Can you work these out from the model? Positions are in its coordinate system, mm. A direction names the side the tool comes from. Coordinates: 2 decimals unless noted, no trailing zeros. Order: outer loops, then holes, each group sorted by start corner. A loop starts at its lowest first (then second) coordinate and runs counter-clockwise, first axis right, second up. Notation, with made-up numbers: (13.5, 12) -> (24.5, 12) arc R14 cw to (24.5, 25) -> close; hole circle Ø10 at (38, 40). An arc over 180 degrees is marked (long way). Use a Markdown table: item, result. Add a question column.
1. For faces 1 (the flat face through (6.4, -3.64, 3.92)), 2 (the conical face through (0.02, 4.89, 4.49)), 3 (the conical face through (-0.02, 4.89, 1.49)), which set-ups out of +Z, -Z, +X, -X, +Y, -Y let a thin tool reach every point of the face, with its end or its side?
2. For pin 1 Ø5 at (y, z) = (-4, 16.5) entering from +X; pin 2 Ø1.5 at (y, z) = (5, 9.5) entering from -X; pin 3 Ø1 at (x, y) = (-1, 0.5) entering from -Z; pin 4 Ø5 at (x, y) = (2.5, -3.5) entering from -Z, each with a flat end and sliding along its axis, tell me the tip position at first contact or that it passes through.
3. We'd pull the mould along Y, two halves only. Please class faces 4 (the conical face through (0.02, 4.89, 2.99)), 5 (the cylindrical face through (-3.988, 6.935, 3.749)), 6 (the cylindrical face through (-8, 0, 4)), 7 (the conical face through (0.02, 4.91, 4.97)): pulls with the +Y half, pulls with the -Y half, needs draft (parallel to the pull), parting line crosses it, or undercut.
4. If I drill on line 1 along X through (y, z) = (0, 5.75); line 2 along Z through (x, y) = (-4.75, 0.5); line 3 along X through (y, z) = (0, 2.65), over which ranges is the centre line in solid material (lowest first)? Write a range as from..to.
5. Suppose I cut it at B-B, the plane z = 12.5. List the corners of the cut face in (x, y) for me, then the cut area to 3 significant figures.
6. Suppose I cut it at A-A, the plane z = 5.5. List the corners of the cut face in (x, y) for me.
```python
from build123d import *

# Parameters (mm, degrees)
SKETCH001_R         = 14.291544
POCKET_DEPTH        = 24.501
REVOLUTION001_ANGLE = 30
REVOLUTION002_ANGLE = 30
REVOLUTION003_ANGLE = 30
REVOLUTION004_ANGLE = 30


with BuildPart() as part:
    # Sketch → Revolution (revolve)
    with BuildSketch(Plane.XZ):
        with BuildLine():
            Line((-5.3, 0), (-5.3, 6))
            ThreePointArc((-5.3, 6), (-4.244457, 6.413224), (-3.75, 7.433241))
            Line((-3.75, 7.433241), (-3, 17))
            Line((-3, 17), (-1.75, 20.5))
            Line((-1.75, 20.5), (-1.25, 20.5))
            Line((-1.25, 20.5), (-0.4, 24.5))
            Line((-0.4, 24.5), (-0.6, 24.5))
            Line((-5.526565, 16.862743), (-0.6, 24.5))
            Line((-5.526565, 16.862743), (-6.174059, 8.578152))
            Line((-6.174059, 8.578152), (-8, 7.60349))
            Line((-8, 7.60349), (-8, 0))
            Line((-5.3, 0), (-8, 0))
        make_face()
    revolve(axis=Axis((0, 0, 0), (0, 0, 1)))

    # Sketch001 (on Face12 of Revolution) → Pocket (cut, through all)
    with BuildSketch(Plane(origin=(0, 0, 0), x_dir=(1, 0, 0), z_dir=(0, 0, -1))):
        Circle(SKETCH001_R)
        Polygon((8.5, 0), (4.25, 7.361216), (-4.25, 7.361216), (-8.5, 0), (-4.25, -7.361216), (4.25, -7.361216), align=None, mode=Mode.SUBTRACT)
    extrude(amount=-POCKET_DEPTH, mode=Mode.SUBTRACT)

    # Sketch002 → Revolution001 (revolve, symmetric)
    with BuildSketch(Plane.XZ) as revolution001_sk:
        Polygon((-5.5, 0), (-4.5, 0.6), (-5.5, 1.2), (-6.5, 1.2), (-6.5, 0), align=None)
        Polygon((-5.5, 1.5), (-4.5, 2.1), (-5.5, 2.7), (-6.5, 2.7), (-6.5, 1.5), align=None)
        Polygon((-5.5, 3), (-4.5, 3.6), (-5.5, 4.2), (-6.5, 4.2), (-6.5, 3), align=None)
    revolve(axis=Axis((0, 0, 0), (0, 0, 1)), revolution_arc=REVOLUTION001_ANGLE / 2)
    revolve(revolution001_sk.sketch, axis=Axis((0, 0, 0), (0, 0, -1)), revolution_arc=REVOLUTION001_ANGLE / 2)

    # Sketch003 → Revolution002 (revolve, symmetric)
    with BuildSketch(Plane(origin=(0, 0, 0.375), x_dir=(0, 1, 0), z_dir=(1, 0, 0))) as revolution002_sk:
        Polygon((-5.5, 0), (-4.5, 0.6), (-5.5, 1.2), (-6.5, 1.2), (-6.5, 0), align=None)
        Polygon((-5.5, 1.5), (-4.5, 2.1), (-5.5, 2.7), (-6.5, 2.7), (-6.5, 1.5), align=None)
        Polygon((-5.5, 3), (-4.5, 3.6), (-5.5, 4.2), (-6.5, 4.2), (-6.5, 3), align=None)
    revolve(axis=Axis((0, 0, 0.375), (0, 0, 1)), revolution_arc=REVOLUTION002_ANGLE / 2)
    revolve(revolution002_sk.sketch, axis=Axis((0, 0, 0.375), (0, 0, -1)), revolution_arc=REVOLUTION002_ANGLE / 2)

    # Sketch004 → Revolution003 (revolve, symmetric)
    with BuildSketch(Plane(origin=(0, 0, 0.75), x_dir=(-1, 0, 0), z_dir=(0, 1, 0))) as revolution003_sk:
        Polygon((-5.5, 0), (-4.5, 0.6), (-5.5, 1.2), (-6.5, 1.2), (-6.5, 0), align=None)
        Polygon((-5.5, 1.5), (-4.5, 2.1), (-5.5, 2.7), (-6.5, 2.7), (-6.5, 1.5), align=None)
        Polygon((-5.5, 3), (-4.5, 3.6), (-5.5, 4.2), (-6.5, 4.2), (-6.5, 3), align=None)
    revolve(axis=Axis((0, 0, 0.75), (0, 0, 1)), revolution_arc=REVOLUTION003_ANGLE / 2)
    revolve(revolution003_sk.sketch, axis=Axis((0, 0, 0.75), (0, 0, -1)), revolution_arc=REVOLUTION003_ANGLE / 2)

    # Sketch005 → Revolution004 (revolve, symmetric)
    with BuildSketch(Plane(origin=(0, 0, 1.125), x_dir=(0, -1, 0), z_dir=(-1, 0, 0))) as revolution004_sk:
        Polygon((-5.5, 0), (-4.5, 0.6), (-5.5, 1.2), (-6.5, 1.2), (-6.5, 0), align=None)
        Polygon((-5.5, 1.5), (-4.5, 2.1), (-5.5, 2.7), (-6.5, 2.7), (-6.5, 1.5), align=None)
        Polygon((-5.5, 3), (-4.5, 3.6), (-5.5, 4.2), (-6.5, 4.2), (-6.5, 3), align=None)
    revolve(axis=Axis((0, 0, 1.125), (0, 0, 1)), revolution_arc=REVOLUTION004_ANGLE / 2)
    revolve(revolution004_sk.sketch, axis=Axis((0, 0, 1.125), (0, 0, -1)), revolution_arc=REVOLUTION004_ANGLE / 2)


solid = part.part
```
Worked out:
| question | item | result |
|---|---|---|
| 1 | face 1 | +Z, -Z, +X, -Y |
| 1 | face 2 | none |
| 1 | face 3 | -Z |
| 2 | pin 1 | stops at x = 5.38 |
| 2 | pin 2 | stops at x = -4.38 |
| 2 | pin 3 | stops at z = 20.5 |
| 2 | pin 4 | stops at z = 0 |
| 3 | face 4 | undercut |
| 3 | face 5 | pulls with the +Y half |
| 3 | face 6 | parting line crosses it |
| 3 | face 7 | undercut |
| 4 | line 1 | x = -8..-5.3, 5.3..8 |
| 4 | line 2 | z = 0.43..0.77, 1.93..2.27, 3.43..3.77, 6.09..18.03 |
| 4 | line 3 | x = -8..-5.3, 4.83..8 |
| 5 | outline | circle Ø11.74 at (0, 0); hole circle Ø6.71 at (0, 0) |
| 5 | area | 72.8 mm² |
| 6 | outline | (-7.94, -0.97) -> (-4.81, -6.39) arc R8 ccw to (-3.13, -7.36) -> (3.13, -7.36) arc R8 ccw to (4.81, -6.39) -> (7.94, -0.97) arc R8 ccw to (7.94, 0.97) -> (4.81, 6.39) arc R8 ccw to (3.13, 7.36) -> (-3.13, 7.36) arc R8 ccw to (-4.81, 6.39) -> (-7.94, 0.97) arc R8 ccw to start; hole circle Ø10.6 at (0, 0) |
